Print and shaded views of the part. All mm, measured from the part's lowest x, y and z. A direction names the side the tool comes from. Give positions to 0.01 mm unless a question says otherwise; leave off trailing zeros. Order: outer loops, then holes, each group sorted by start corner. A loop starts at its lowest first (then second) coordinate and runs counter-clockwise, first axis right, second up. Notation, with made-up numbers: (86.25, -17) - (112.25, -17) arc R15 cw to (112.25, 6) - close; hole circle Ø1 at (74.5, -12). An arc over 180 degrees is marked (long way). Answer in a Markdown table with one row per item.
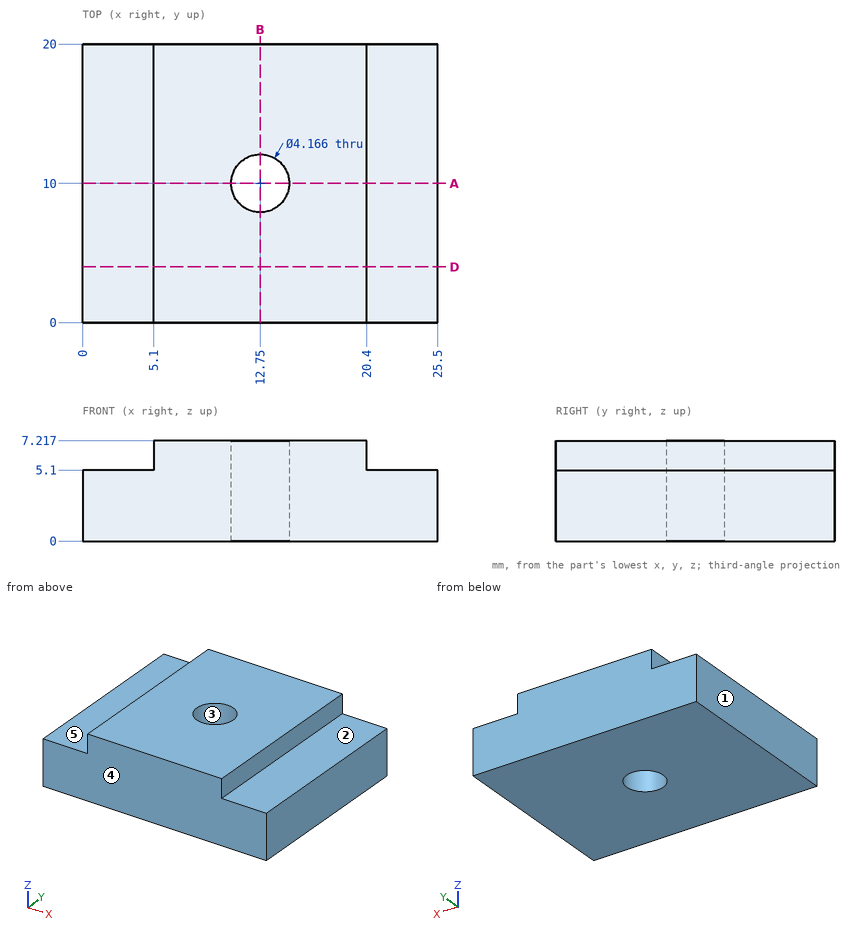
1. Which spindle directions (+Z, -Z, +X, -X, +Y, -Y) get a long thin tool onto all of the face, cutting with end or side? Do the marked faces 1 and 2. Say none if no direction does.
Check result:
| item | result |
|---|---|
| face 1 | +Z, -Z, -X, +Y, -Y |
| face 2 | +Z, +X, +Y, -Y |
2. Drop flat-ended pins along their axis: P1, Ø2.5, axis at x = 2, y = 6, coming from the +Z side; P2, Ø1.7, axis at y = 5.5, z = 6.5, coming from the -X side; P3, Ø2.5, axis at y = 8.5, z = 6.5, coming from the +X side. Give the stop position or say it passes through.
Check result:
| item | result |
|---|---|
| P1 | stops at z = 5.1 |
| P2 | stops at x = 5.1 |
| P3 | stops at x = 20.4 |
3. Cut at B-B on x = 12.75. Write the cut outline in (y, z), and give its area (3 significant figures).
Check result:
| item | result |
|---|---|
| outline | (0, 0) - (7.92, 0) - (7.92, 7.22) - (0, 7.22) - close; (12.08, 0) - (20, 0) - (20, 7.22) - (12.08, 7.22) - close |
| area | 114 mm² |
4. Cut at A-A on y = 10. Write the cut outline in (x, z), and give its area (3 significant figures).
Check result:
| item | result |
|---|---|
| outline | (0, 0) - (10.67, 0) - (10.67, 7.22) - (5.1, 7.22) - (5.1, 5.1) - (0, 5.1) - close; (14.83, 0) - (25.5, 0) - (25.5, 5.1) - (20.4, 5.1) - (20.4, 7.22) - (14.83, 7.22) - close |
| area | 132 mm² |
5. Two-plate mould, pull along Y, no slides. Class the marked faces 3, 4 and 5: +Y half, -Y half, draft (parallel to the pull), parting line (faces both ways), or undercut.
Check result:
| item | result |
|---|---|
| face 3 | undercut |
| face 4 | -Y half |
| face 5 | draft |
6. Cut at D-D on y = 4. Write the cut outline in (x, z).
Check result:
| item | result |
|---|---|
| outline | (0, 0) - (25.5, 0) - (25.5, 5.1) - (20.4, 5.1) - (20.4, 7.22) - (5.1, 7.22) - (5.1, 5.1) - (0, 5.1) - close |
7. Probe line 1 (Y direction, x = 12.75, z = 3); line 2 (Z direction, x = 22, y = 8.75); line 3 (X direction, y = 15, z = 5.5). List the from-to ranges inside material, lowest first.
Check result:
| item | result |
|---|---|
| line 1 | y = 0 to 7.92, 12.08 to 20 |
| line 2 | z = 0 to 5.1 |
| line 3 | x = 5.1 to 20.4 |
